Geometry: final body of the model. Coordinates: model frame, mm. Face numbers are marked on the shaded views. A direction names the side the tool comes from. Coordinates: 2 decimals unless noted, no trailing zeros. Write each loop counter-clockwise with the first axis right and the second up, starting at its lowest first coordinate (ties: lowest second). Pieces come first, ordered by that corner, then holes. Notation, with made-up numbers: (-32, 15.25) - (-27, 15.25) arc R28 cw to (-27, 35.25) - close; hole circle Ø5 at (25, 52). An arc over 180 degrees is marked (long way). Put each result on its own line as item: value.
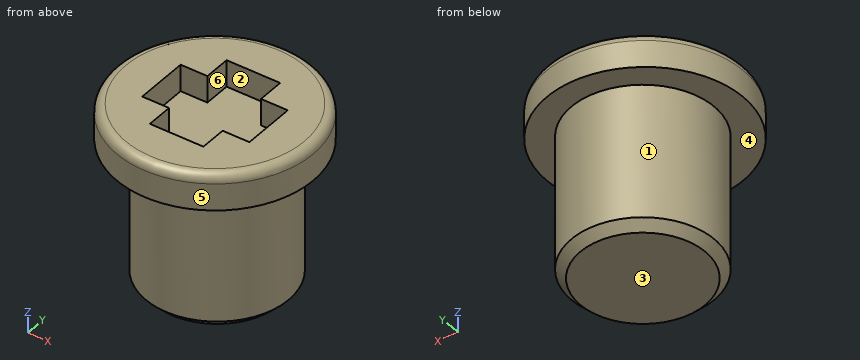
```python
from build123d import *

# Parameters (mm, degrees)
SKETCH1_R           = 4
BOSS_EXTRUDE1_DEPTH = 8
SKETCH2_R           = 5.5
BOSS_EXTRUDE2_DEPTH = 2
CHAMFER1_SIZE       = 0.5
CUT_EXTRUDE1_DEPTH  = 1.5
FILLET1_R           = 0.5


with BuildPart() as part:
    # Sketch1 → Boss-Extrude1 (new body)
    with BuildSketch(Plane.XY):
        with Locations((0, 0.169439546)):
            Circle(SKETCH1_R)
    extrude(amount=BOSS_EXTRUDE1_DEPTH)

    # Sketch2 → Boss-Extrude2 (add)
    with BuildSketch(Plane.XY.offset(8)):
        Circle(SKETCH2_R)
    extrude(amount=BOSS_EXTRUDE2_DEPTH)

    # Chamfer1
    chamfer1_edges = [part.edges().sort_by_distance(p)[0] for p in [
        (-4, 0.169439546, 0),
    ]]
    chamfer(chamfer1_edges, length=CHAMFER1_SIZE)

    # Sketch4 → Cut-Extrude1 (cut)
    with BuildSketch(Plane.XY.offset(10)):
        Polygon((1.5, 1.5), (3, 1.5), (3, -1.50088727), (1.5, -1.50088727), (1.5, -3), (-1.5, -3), (-1.5, -1.50088727), (-3, -1.50088727), (-3, 0), (-3, 1.5), (-1.5, 1.5), (-1.5, 3), (0, 3), (1.5, 3), align=None)
    extrude(amount=-CUT_EXTRUDE1_DEPTH, mode=Mode.SUBTRACT)

    # Fillet1
    fillet1_edges = [part.edges().sort_by_distance(p)[0] for p in [
        (-5.5, 0, 10),
    ]]
    fillet(fillet1_edges, radius=FILLET1_R)


solid = part.part
```
1. Ray query, probe 1 along Z at (x, y) = (-1, -0.5); probe 2 along Z at (x, y) = (4, -1); probe 3 along X at (y, z) = (3.5, 3.75). Return the intervals inside material, ascending. Write a range as from..to.
Answer below:
probe 1: z = 0..8.5
probe 2: z = 8..10
probe 3: x = -2.22..2.22
2. Section query C-C (z = 1.5). Return loops of the section in (x, y).
Answer below:
outline: circle Ø8 at (0, 0.17)
3. Pin query (flat end, axial travel): pin 1 Ø2 at (y, z) = (3, 2.5) entering from +X; pin 2 Ø0.7 at (y, z) = (-2, 9) entering from +X; pin 3 Ø1.6 at (y, z) = (2.5, 9) entering from -X. Return the tip coordinate at first contact, or that it passes through.
Answer below:
pin 1: stops at x = 3.56
pin 2: stops at x = 5.25
pin 3: stops at x = -5.23
4. Section query B-B (x = 0). Return loops of the section in (y, z), then the cut area to 3 significant figures.
Answer below:
outline: (-5.5, 8) - (-3.83, 8) - (-3.83, 0.5) - (-3.33, 0) - (3.67, 0) - (4.17, 0.5) - (4.17, 8) - (5.5, 8) - (5.5, 9.5) arc R0.5 ccw to (5, 10) - (3, 10) - (3, 8.5) - (-3, 8.5) - (-3, 10) - (-5, 10) arc R0.5 ccw to (-5.5, 9.5) - close
area: 76.6 mm²
5. Set-up query: the marked faces 4, 5 and 6. Return all of +Z, -Z, +X, -X, +Y, -Y with unobstructed straight access to the full face (end or side cutting, diameter ignored); none if empty.
Answer below:
face 4: -Z
face 5: +Z, -Z
face 6: +Z
6. Section query A-A (z = 9). Return loops of the section in (x, y), then the cut area to 3 significant figures.
Answer below:
outline: circle Ø11 at (0, 0); hole (-3, -1.5) - (-1.5, -1.5) - (-1.5, -3) - (1.5, -3) - (1.5, -1.5) - (3, -1.5) - (3, 1.5) - (1.5, 1.5) - (1.5, 3) - (-1.5, 3) - (-1.5, 1.5) - (-3, 1.5) - close
area: 68.0 mm²
7. Mould query, pull axis Y, two halves, no side actions, for the marked faces 1, 2 and 3. Classes: +Y half, -Y half, draft (parallel to the pull), parting line (faces both ways), or undercut.
Answer below:
face 1: parting line
face 2: undercut
face 3: draft
